Check sheet for the modelled part. Datum: model origin and axes. Units: mm. Round coordinates to 2 decimals unless told otherwise and drop trailing zeros. Write each loop counter-clockwise with the first axis right and the second up, starting at its lowest first coordinate (ties: lowest second). Pieces come first, ordered by that corner, then holes.
Item 1: Cross-section at A-A on y = 105. Enter the section's corners in (x, z), plus the area to 3 significant figures.
Item 2: Material ranges on line 1 (X direction, y = 49, z = 4); line 2 (X direction, y = -2.5, z = 2.5); line 3 (Y direction, x = -45, z = 7.5), recorded low to high.
Item 3: Release check for a two-part mould opening along Y. For faces 1 (the flat face through (-2, 125, 5)), 2 (the flat face through (-2, 57, 0)), 3 (the cylindrical face through (-50.957, 46.182, 5.07)) record: +Y half, -Y half, draft (parallel to the pull), parting line (faces both ways), or undercut.
Item 4: Cross-section at C-C on x = 0. Enter the section's corners in (y, z).
from build123d import *

# Parameters (mm, degrees)
F0_W            = 250
F0_H            = 250
F0_R            = 55.5
F1_DEPTH        = 10
F2_R            = 5
F3_DEPTH        = 25
F3_COPIES_COUNT = 4
F4_R            = 6
F5_DEPTH        = 10.001


# Not quite as in the source:
# - a pattern or mirror of a feature is missing from the dataset's text; its kind, count and spacing are read off the source's solid


with BuildPart() as f1:
    # F0 (on Top) → F1 (new body)
    with BuildSketch(Plane.XY):
        Rectangle(F0_W, F0_H)
        Circle(F0_R, mode=Mode.SUBTRACT)
    extrude(amount=F1_DEPTH)

    # F2 (on face) → F3 (cut)
    with BuildSketch(Plane.XY.offset(10)):
        with Locations((-45.9619407771, 45.9619407771)):
            Circle(F2_R)
    f3 = extrude(amount=-F3_DEPTH, mode=Mode.SUBTRACT)

    # F3_copies: F3 ×4 about axis
    f3_copies_axis = Axis((0, 0, 0), (0, 0, 1))
    for i in range(1, F3_COPIES_COUNT):
        add(f3.rotate(f3_copies_axis, i * 360 / F3_COPIES_COUNT), mode=Mode.SUBTRACT)

    # F4 (on face) → F5 (cut, through all)
    with BuildSketch(Plane.XY.offset(10)):
        with Locations((-105, 105)):
            Circle(F4_R)
        with Locations((105, 105)):
            Circle(F4_R)
        with Locations((105, -105)):
            Circle(F4_R)
        with Locations((-105, -105)):
            Circle(F4_R)
    extrude(amount=-F5_DEPTH, mode=Mode.SUBTRACT)


solid = f1.part
Response values:
1. outline: (-125, 0) - (-111, 0) - (-111, 10) - (-125, 10) - close; (-99, 0) - (99, 0) - (99, 10) - (-99, 10) - close; (111, 0) - (125, 0) - (125, 10) - (111, 10) - close
1. area: 2,260 mm2
2. line 1: x = -125 to -49.93, -41.99 to -26.06, 26.06 to 41.99, 49.93 to 125
2. line 2: x = -125 to -55.44, 55.44 to 125
2. line 3: y = -125 to -50.87, -41.06 to -32.48, 32.48 to 41.06, 50.87 to 125
3. face 1: +Y half
3. face 2: draft
3. face 3: undercut
4. outline: (-125, 0) - (-55.5, 0) - (-55.5, 10) - (-125, 10) - close; (55.5, 0) - (125, 0) - (125, 10) - (55.5, 10) - close
